Geometry: final body of the model. Coordinates: model frame, mm. Face numbers are marked on the shaded views. Round coordinates to 2 decimals unless told otherwise and drop trailing zeros. Loops run counter-clockwise (first coordinate to the right, second up) from the corner with the lowest first, then second, coordinate; pieces in that order, holes last. Notation, with made-up numbers: (-13, -15) - (33, -15) arc R23 ccw to (33, -2) - close; hole circle Ø4 at (74.25, -34.5). An arc over 180 degrees is marked (long way). Use CSV: the item, a comma, the result in double quotes.
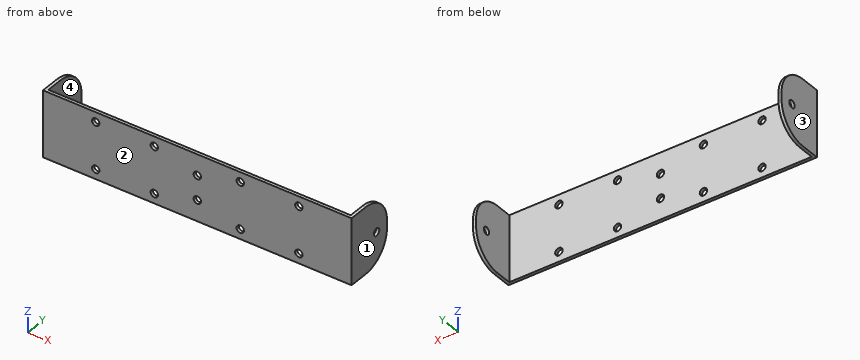
from build123d import *

# Parameters (mm, degrees)
BOSS_EXTRUDE1_DEPTH   = 33.85
F_6_CLEARANCE_HOLE1_D = 3.7973
F_6_CLEARANCE_HOLE2_D = 3.7973
FILLET1_R             = 15
FILLET1_OF_MIRROR1_R  = 15
F_6_CLEARANCE_HOLE3_D = 3.7973


with BuildPart() as part:
    # Sketch1 → Boss-Extrude1 (new body)
    with BuildSketch(Plane.XY):
        Polygon((0, 0), (-79, 0), (-79, 25), (-77.4125, 25), (-77.4125, 1.5875), (0, 1.5875), align=None)
    boss_extrude1 = extrude(amount=BOSS_EXTRUDE1_DEPTH)

    # #6 Clearance Hole1 (through all)
    with Locations(Plane.ZY.offset(79)):
        with Locations((16.925, 17.6675)):
            f_6_clearance_hole1 = Hole(F_6_CLEARANCE_HOLE1_D / 2)

    # #6 Clearance Hole2 (through all)
    with Locations(Plane(origin=(0, 0, 0), x_dir=(-1, 0, 0), z_dir=(0, -1, 0))):
        with Locations((22, -5), (52, -5), (52, -28.85), (22, -28.85)):
            f_6_clearance_hole2 = Hole(F_6_CLEARANCE_HOLE2_D / 2)

    # Fillet1
    fillet1_edges = [part.edges().sort_by_distance(p)[0] for p in [
        (-78.20625, 25, 33.85),
        (-78.20625, 25, 0),
    ]]
    fillet(fillet1_edges, radius=FILLET1_R)

    # Mirror1: Boss-Extrude1, #6 Clearance Hole1, #6 Clearance Hole2 across plane
    add(boss_extrude1.mirror(Plane(origin=(0, 0, 0), x_dir=(0, 0, 1), z_dir=(1, 0, 0))))
    add(f_6_clearance_hole1.mirror(Plane(origin=(0, 0, 0), x_dir=(0, 0, 1), z_dir=(1, 0, 0))), mode=Mode.SUBTRACT)
    add(f_6_clearance_hole2.mirror(Plane(origin=(0, 0, 0), x_dir=(0, 0, 1), z_dir=(1, 0, 0))), mode=Mode.SUBTRACT)

    # Fillet1 of Mirror1
    fillet1_of_mirror1_edges = [part.edges().sort_by_distance(p)[0] for p in [
        (78.20625, 25, 33.85),
        (78.20625, 25, 0),
    ]]
    fillet(fillet1_of_mirror1_edges, radius=FILLET1_OF_MIRROR1_R)

    # #6 Clearance Hole3 (through all)
    with Locations(Plane(origin=(0, 0, 0), x_dir=(-1, 0, 0), z_dir=(0, -1, 0))):
        with Locations((0, -23.125), (0, -10.725)):
            Hole(F_6_CLEARANCE_HOLE3_D / 2)


solid = part.part
Item 1: Section D-D on x = 3.5. Return the cut outline in (y, z), plus the area to 3 significant figures.
Final values:
outline,"(0, 0) - (1.59, 0) - (1.59, 33.85) - (0, 33.85) - close"
area,"53.7 mm²"
Item 2: Section A-A on x = 22. Return the cut outline in (y, z).
Final values:
outline,"(0, 0) - (1.59, 0) - (1.59, 3.1) - (0, 3.1) - close; (0, 6.9) - (1.59, 6.9) - (1.59, 26.95) - (0, 26.95) - close; (0, 30.75) - (1.59, 30.75) - (1.59, 33.85) - (0, 33.85) - close"
Item 3: Section C-C on y = 23.5. Return the cut outline in (x, z).
Final values:
outline,"(-79, 8.46) - (-77.41, 8.46) - (-77.41, 25.39) - (-79, 25.39) - close; (77.41, 8.46) - (79, 8.46) - (79, 25.39) - (77.41, 25.39) - close"
Item 4: Pin query (flat end, axial travel): P1, Ø5, axis at x = -47, z = 9.5, coming from the +Y side; P2, Ø8, axis at x = -59.5, y = 5, coming from the -Z side. Return the tip coordinate at first contact, or that it passes through.
Final values:
P1,"stops at y = 1.59"
P2,"stops at z = 0"
Item 5: Mould query, pull axis X, two halves, no side actions, for the marked faces 1, 2, 3 and 4. Classes: released by +X, released by -X, zero draft, split by the parting line, or undercut.
Final values:
face 1,"released by +X"
face 2,"zero draft"
face 3,"released by -X"
face 4,"undercut"
Item 6: Material intervals for line 1 (Z direction, x = -22, y = 1.25); line 2 (Z direction, x = 0, y = 0.6); line 3 (X direction, y = 3, z = 25), sorted ascending.
Final values:
line 1,"z = 0 to 3.1, 6.9 to 26.95, 30.75 to 33.85"
line 2,"z = 0 to 8.83, 12.62 to 21.23, 25.02 to 33.85"
line 3,"x = -79 to -77.41, 77.41 to 79"
Item 7: Section B-B on z = 5. Return the cut outline in (x, y), plus the area to 3 significant figures.
Final values:
outline,"(-79, 0) - (-53.9, 0) - (-53.9, 1.59) - (-77.41, 1.59) - (-77.41, 21.18) - (-79, 21.18) - close; (-50.1, 0) - (-23.9, 0) - (-23.9, 1.59) - (-50.1, 1.59) - close; (-20.1, 0) - (20.1, 0) - (20.1, 1.59) - (-20.1, 1.59) - close; (23.9, 0) - (50.1, 0) - (50.1, 1.59) - (23.9, 1.59) - close; (53.9, 0) - (79, 0) - (79, 21.18) - (77.41, 21.18) - (77.41, 1.59) - (53.9, 1.59) - close"
area,"289 mm²"
